Check sheet for the drawn part. Datum: minimum x, y, z corner. Units: mm. Coordinates: 2 decimals unless noted, no trailing zeros. Write each loop counter-clockwise with the first axis right and the second up, starting at its lowest first coordinate (ties: lowest second). Pieces come first, ordered by that corner, then holes. Notation, with made-up numbers: (35, -32) -> (87, -32) arc R17 ccw to (87, -12) -> close; hole circle Ø2 at (-3.75, -8). An arc over 180 degrees is marked (long way). Answer in a Markdown table with one row per item.
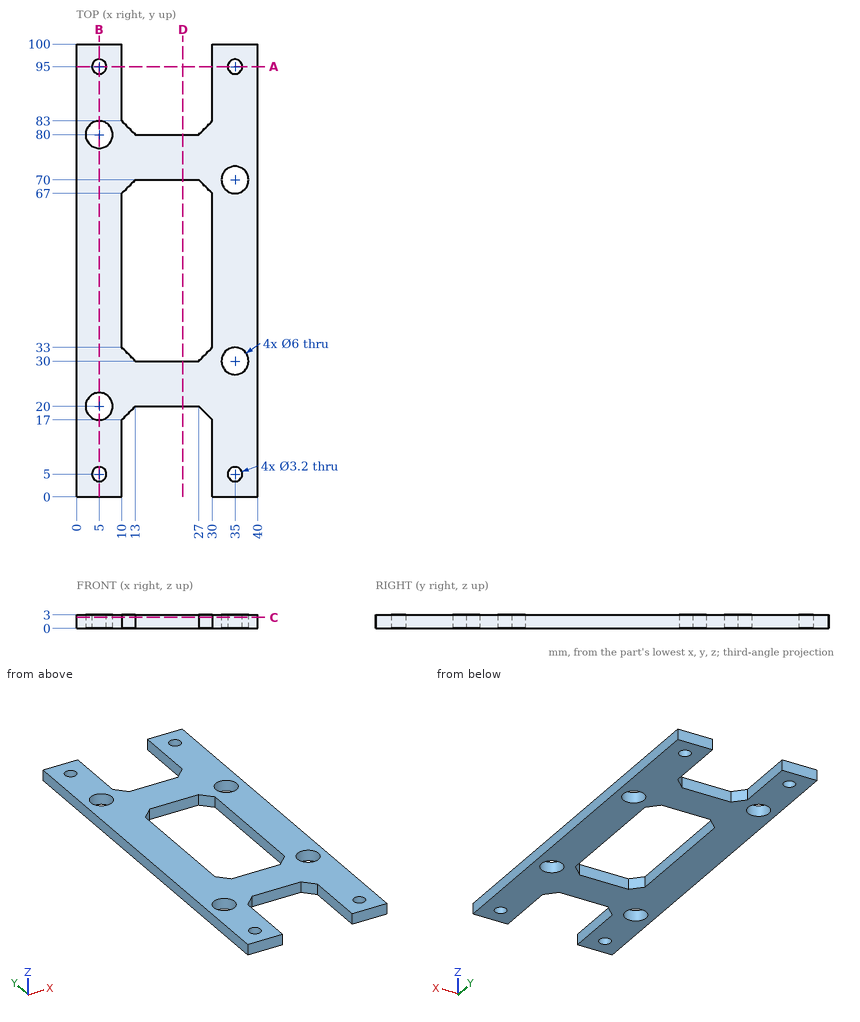
1. Sectioned sample at A-A, the plane y = 95. Record the cut outline in (x, z), and give its area (3 significant figures).
Findings below:
| item | result |
|---|---|
| outline | (0, 0) -> (3.4, 0) -> (3.4, 3) -> (0, 3) -> close; (6.6, 0) -> (10, 0) -> (10, 3) -> (6.6, 3) -> close; (30, 0) -> (33.4, 0) -> (33.4, 3) -> (30, 3) -> close; (36.6, 0) -> (40, 0) -> (40, 3) -> (36.6, 3) -> close |
| area | 40.8 mm² |
2. Material ranges on probe 1 along Y at (x, z) = (5, 1.15); probe 2 along Y at (x, z) = (35, 1.9); probe 3 along X at (y, z) = (95, 1.75), recorded low to high. Write a range as from..to.
Findings below:
| item | result |
|---|---|
| probe 1 | y = 0..3.4, 6.6..17, 23..77, 83..93.4, 96.6..100 |
| probe 2 | y = 0..3.4, 6.6..27, 33..67, 73..93.4, 96.6..100 |
| probe 3 | x = 0..3.4, 6.6..10, 30..33.4, 36.6..40 |
3. Sectioned sample at D-D, the plane x = 23.5. Record the cut outline in (y, z), and give its area (3 significant figures).
Findings below:
| item | result |
|---|---|
| outline | (20, 0) -> (30, 0) -> (30, 3) -> (20, 3) -> close; (70, 0) -> (80, 0) -> (80, 3) -> (70, 3) -> close |
| area | 60.0 mm² |
4. Sectioned sample at B-B, the plane x = 5. Record the cut outline in (y, z), and give its area (3 significant figures).
Findings below:
| item | result |
|---|---|
| outline | (0, 0) -> (3.4, 0) -> (3.4, 3) -> (0, 3) -> close; (6.6, 0) -> (17, 0) -> (17, 3) -> (6.6, 3) -> close; (23, 0) -> (77, 0) -> (77, 3) -> (23, 3) -> close; (83, 0) -> (93.4, 0) -> (93.4, 3) -> (83, 3) -> close; (96.6, 0) -> (100, 0) -> (100, 3) -> (96.6, 3) -> close |
| area | 245 mm² |
5. Sectioned sample at C-C, the plane z = 2.45. Count the separate pieces of the cut face and the enclosed holes in it, and give its area (3 significant figures).
Findings below:
| item | result |
|---|---|
| separate pieces | 1 |
| enclosed holes | 9 |
| area | 2,290 mm² |
6. Go/stop test with flat-tipped pins: pin 1 (10 mm diameter, centred on x = 19.5, y = 47.5, fed in from +Z); pin 2 (5 mm diameter, centred on x = 5, y = 5, fed in from +Z); pin 3 (1.5 mm diameter, centred on x = 11.5, z = 1, fed in from +Y); pin 4 (0.9 mm diameter, centred on x = 20.5, z = 2, fed in from +Y). Record where each tip stops, or that it passes through.
Findings below:
| item | result |
|---|---|
| pin 1 | passes through |
| pin 2 | stops at z = 3 |
| pin 3 | stops at y = 82.25 |
| pin 4 | stops at y = 80 |
